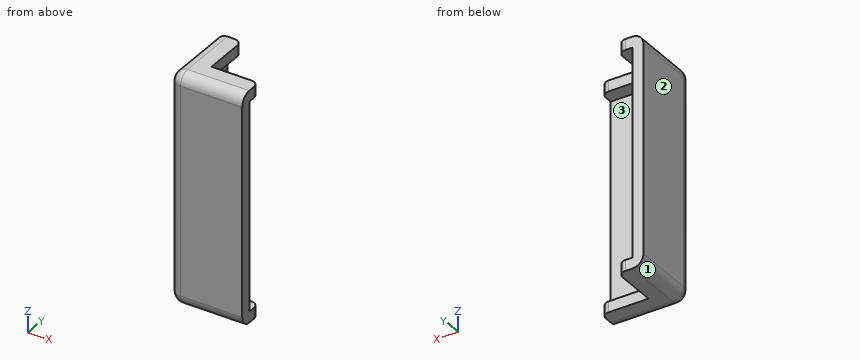
from build123d import *

# Parameters (mm, degrees)
PAD_DEPTH    = 63.4
SKETCH001_W  = 20
SKETCH001_H  = 20
POCKET_DEPTH = 57.4
FILLET_R     = 2
FILLET001_R  = 3


with BuildPart() as part:
    # Sketch → Pad (new body)
    with BuildSketch(Plane.XY):
        Polygon((0, 0), (20, 0), (20, 7), (7, 7), (7, 20), (0, 20), align=None)
    extrude(amount=PAD_DEPTH)

    # Sketch001 (on DatumPlane) → Pocket (cut)
    with BuildSketch(Plane(origin=(0, 0, 3), x_dir=(-1, 0, 0), z_dir=(0, 0, 1))):
        with Locations((-13, -13)):
            Rectangle(SKETCH001_W, SKETCH001_H)
    extrude(amount=POCKET_DEPTH, mode=Mode.SUBTRACT)

    # Fillet
    fillet_edges = [part.edges().sort_by_distance(p)[0] for p in [
        (7, 20, 61.9),
        (20, 7, 61.9),
        (7, 20, 1.5),
        (20, 7, 1.5),
    ]]
    fillet(fillet_edges, radius=FILLET_R)

    # Fillet001
    fillet001_edges = [part.edges().sort_by_distance(p)[0] for p in [
        (10, 0, 63.4),
        (0, 10, 63.4),
        (0, 0, 31.7),
        (0, 10, 0),
        (10, 0, 0),
    ]]
    fillet(fillet001_edges, radius=FILLET001_R)


solid = part.part
Source: CAD feature listing. Evaluate the final solid. Frame: model axes, mm. Face numbers are marked on the shaded views. Give positions to 0.01 mm unless a question says otherwise; leave off trailing zeros. Write each loop counter-clockwise with the first axis right and the second up, starting at its lowest first coordinate (ties: lowest second). Pieces come first, ordered by that corner, then holes. Notation, with made-up numbers: (43, 82.5) -> (62, 82.5) arc R6 ccw to (62, 87.5) -> close; hole circle Ø5 at (37, 63). An arc over 180 degrees is marked (long way). Write item = value, one per line.
Q1. Cut plane B-B on x = 10. Return loops of the section in (y, z), then the cut area to 3 significant figures.
Here are the results:
outline = (0, 3) arc R3 ccw to (3, 0) -> (7, 0) -> (7, 3) -> (3, 3) -> (3, 60.4) -> (7, 60.4) -> (7, 63.4) -> (3, 63.4) arc R3 ccw to (0, 60.4) -> close
area = 210 mm²
Q2. Line query: line 1 (Z direction, x = 5, y = 5.25); line 2 (Y direction, x = 2.75, z = 21); line 3 (X direction, y = 18.25, z = 44.5). Output: solid intervals per line, ascending. Write a range as from..to.
Here are the results:
line_1 = 0..3, 60.4..63.4
line_2 = 0.01..20
line_3 = 0..3
Q3. Mould query, pull axis Z, two halves, no side actions, for the marked faces 1, 2 and 3. Classes: +Z half, -Z half, draft (parallel to the pull), parting line (faces both ways), or undercut.
Here are the results:
face_1 = -Z half
face_2 = draft
face_3 = undercut
Q4. First-contact query: pin 1 (0.9 mm diameter, centred on y = 12.5, z = 1, fed in from +X); pin 2 (1.5 mm diameter, centred on x = 10, z = 62, fed in from +Y); pin 3 (8.5 mm diameter, centred on x = 8.5, z = 32.5, fed in from +Y); pin 4 (5 mm diameter, centred on x = 11, y = 12, fed in from +Z). Flat tips, straight axial feed; report the tip coordinate or a pass-through.
Here are the results:
pin_1 = 7
pin_2 = 7
pin_3 = 3
pin_4 = through
Q5. Cut plane D-D on y = 2. Return loops of the section in (x, z).
Here are the results:
outline = (0.17, 3) arc R2.83 ccw to (3, 0.17) -> (20, 0.17) -> (20, 63.23) -> (3, 63.23) arc R2.83 ccw to (0.17, 60.4) -> close
Q6. Cut plane A-A on z = 59. Return loops of the section in (x, y).
Here are the results:
outline = (0, 3) arc R3 ccw to (3, 0) -> (20, 0) -> (20, 3) -> (3, 3) -> (3, 20) -> (0, 20) -> close
